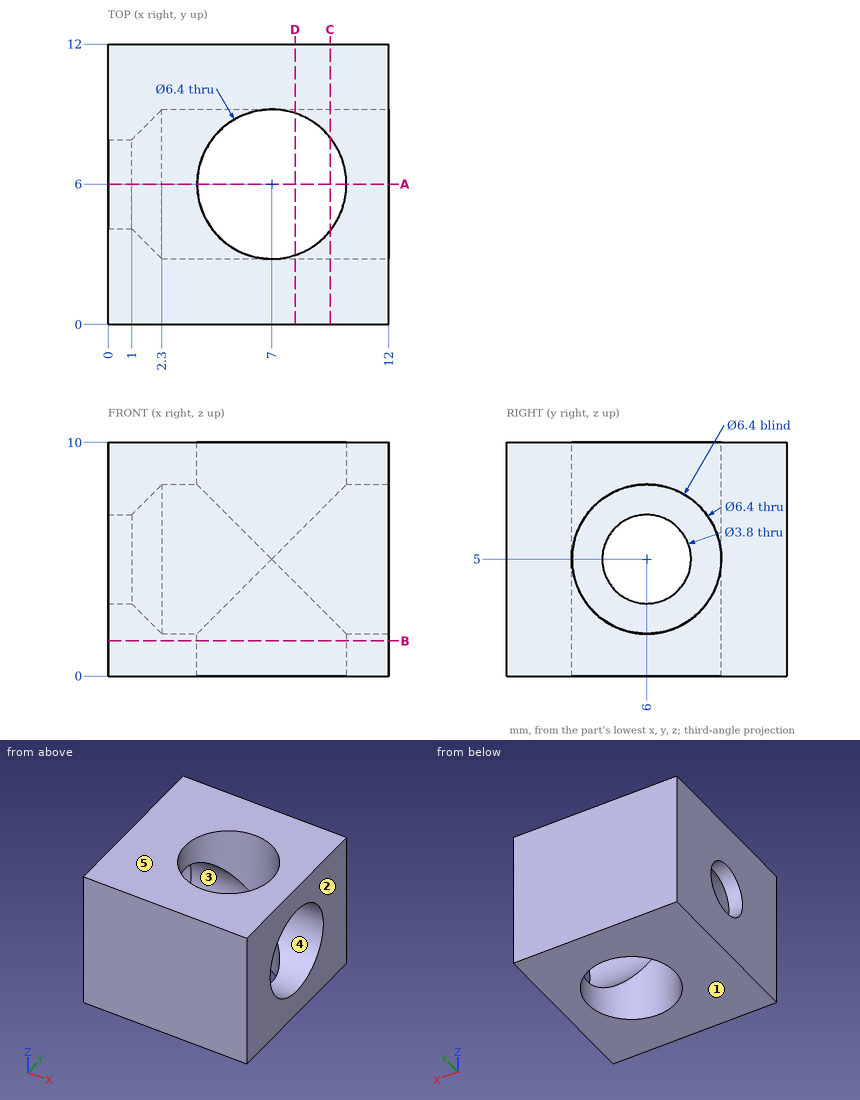
Part print with two shaded views. Sizes in mm from the minimum x, y, z corner. A direction names the side the tool comes from. Round coordinates to 2 decimals unless told otherwise and drop trailing zeros. Order: outer loops, then holes, each group sorted by start corner. A loop starts at its lowest first (then second) coordinate and runs counter-clockwise, first axis right, second up. Notation, with made-up numbers: (8.5, -22) - (23.5, -22) arc R28 cw to (23.5, 12) - close; hole circle Ø7 at (65.25, 17.25). An arc over 180 degrees is marked (long way). Answer in a Markdown table with one row per item. Add a question column.
(1) Drop a flat-ended pin along its axis: pin 1 Ø4 at (x, y) = (7, 6) entering from +Z. Give the stop position or say it passes through.
(2) 3-axis set-ups, long thin cutter, end or side, ignore diameter. For the marked faces 4 and 5: which of +Z, -Z, +X, -X, +Y, -Y reach the whole face in a straight line?
(3) Band-saw the part on D-D on x = 8. List the corners of the cut face in (y, z), and give its area (3 significant figures).
(4) Mould opens along Z. For the marked faces 1, 2 and 3 say: +Z half, -Z half, draft (parallel to the pull), parting line (faces both ways), or undercut.
(5) Band-saw the part on A-A on y = 6. List the corners of the cut face in (x, z).
(6) Band-saw the part on B-B on z = 1.5. List the corners of the cut face in (x, y), and give its area (3 significant figures).
(7) Band-saw the part on C-C on x = 9.5. List the corners of the cut face in (y, z).
(8) Probe L1, parallel to Z at x = 0.25, y = 6; L2, parallel to Y at x = 4.95, z = 5; L3, parallel to Z at x = 3.4, y = 6. List the from-to ranges inside material, lowest first. Write a range as [from, to].
Data:
| question | item | result |
|---|---|---|
| 1 | pin 1 | passes through |
| 2 | face 4 | +X |
| 2 | face 5 | +Z, +X, -X, +Y, -Y |
| 3 | outline | (0, 0) - (2.96, 0) - (2.96, 4) arc R3.2 cw to (2.96, 6) - (2.96, 10) - (0, 10) - close; (9.04, 0) - (12, 0) - (12, 10) - (9.04, 10) - (9.04, 6) arc R3.2 cw to (9.04, 4) - close |
| 3 | area | 58.8 mm^2 |
| 4 | face 1 | -Z half |
| 4 | face 2 | draft |
| 4 | face 3 | undercut |
| 5 | outline | (0, 0) - (3.8, 0) - (3.8, 1.8) - (2.3, 1.8) - (1, 3.1) - (0, 3.1) - close; (0, 6.9) - (1, 6.9) - (2.3, 8.2) - (3.8, 8.2) - (3.8, 10) - (0, 10) - close; (10.2, 0) - (12, 0) - (12, 1.8) - (10.2, 1.8) - close; (10.2, 8.2) - (12, 8.2) - (12, 10) - (10.2, 10) - close |
| 6 | outline | (0, 0) - (12, 0) - (12, 12) - (0, 12) - close; hole circle Ø6.4 at (7, 6) |
| 6 | area | 112 mm^2 |
| 7 | outline | (0, 0) - (4, 0) - (4, 2.5) arc R3.2 cw to (4, 7.5) - (4, 10) - (0, 10) - close; (8, 0) - (12, 0) - (12, 10) - (8, 10) - (8, 7.5) arc R3.2 cw to (8, 2.5) - close |
| 8 | L1 | z = [0, 3.1], [6.9, 10] |
| 8 | L2 | y = [0, 2.8], [9.2, 12] |
| 8 | L3 | z = [0, 1.8], [8.2, 10] |
